Check sheet for the drawn part. Datum: minimum x, y, z corner. Units: mm. A direction names the side the tool comes from. Coordinates: 2 decimals unless noted, no trailing zeros. Loops run counter-clockwise (first coordinate to the right, second up) from the corner with the lowest first, then second, coordinate; pieces in that order, holes last. Notation, with made-up numbers: (17.25, 34.5) -> (42.25, 34.5) arc R23 ccw to (42.25, 61.5) -> close; hole circle Ø1 at (53.5, 41). An arc over 180 degrees is marked (long way). Use CSV: the item, a comma, the result in double quotes. Start each with the question number.
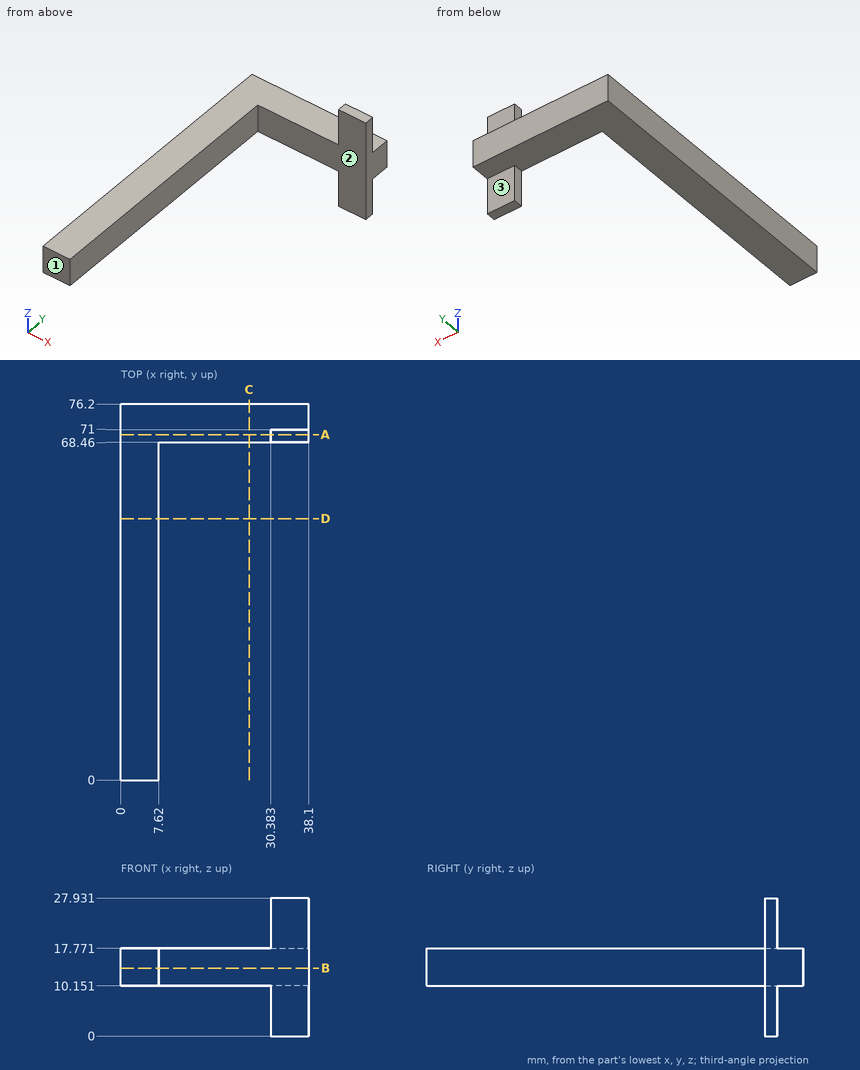
1. Set-up check for the marked faces 1, 2 and 3: record each of +Z, -Z, +X, -X, +Y, -Y from which the full face is reachable in a straight line by a thin tool's end or side.
2. Cross-section at A-A, the plane y = 70. Record the boundary of the cut face in (x, z), plus the area to 3 significant figures.
3. Cross-section at C-C, the plane x = 26. Record the boundary of the cut face in (y, z).
4. Cross-section at D-D, the plane y = 53. Record the boundary of the cut face in (x, z).
5. Cross-section at B-B, the plane z = 13.75. Record the boundary of the cut face in (x, y).
6. Depth check by flat-ended pin: pin 1 (8.5 mm diameter, centred on y = 29, z = 14.5, fed in from +X); pin 2 (0.8 mm diameter, centred on y = 70, z = 5, fed in from -X); pin 3 (5 mm diameter, centred on x = 13, z = 13.5, fed in from -Y). Enter the tip coordinate at first touch or a pass-through.
7. Scan lines: line 1 (Z direction, x = 4.5, y = 62.5); line 2 (Y direction, x = 35, z = 1.25); line 3 (X direction, y = 39, z = 13.25). Record each from-to range of solid material in increasing order.
Solution:
1,face 1,"+Z, -Z, +X, -X, -Y"
1,face 2,"+Z, -Z, +X, -Y"
1,face 3,"-Z, +X, -X, +Y"
2,outline,"(0, 10.15) -> (30.38, 10.15) -> (30.38, 0) -> (38.1, 0) -> (38.1, 27.93) -> (30.38, 27.93) -> (30.38, 17.77) -> (0, 17.77) -> close"
2,area,"447 mm2"
3,outline,"(68.46, 10.15) -> (76.2, 10.15) -> (76.2, 17.77) -> (68.46, 17.77) -> close"
4,outline,"(0, 10.15) -> (7.62, 10.15) -> (7.62, 17.77) -> (0, 17.77) -> close"
5,outline,"(0, 0) -> (7.62, 0) -> (7.62, 68.46) -> (38.1, 68.46) -> (38.1, 76.2) -> (0, 76.2) -> close"
6,pin 1,"stops at x = 7.62"
6,pin 2,"stops at x = 30.38"
6,pin 3,"stops at y = 68.46"
7,line 1,"z = 10.15 to 17.77"
7,line 2,"y = 68.46 to 71"
7,line 3,"x = 0 to 7.62"
